from build123d import *

# Parameters (mm, degrees)
SKETCH1_R           = 10.75
BOSS_EXTRUDE1_DEPTH = 7.1
BOSS_EXTRUDE2_DEPTH = 1.5875
SKETCH3_R           = 2.54
BOSS_EXTRUDE3_DEPTH = 29
FILLET1_R           = 1.27


with BuildPart() as part:
    # Sketch1 → Boss-Extrude1 (new body)
    with BuildSketch(Plane(origin=(0, 0, 0), x_dir=(1, 0, 0), z_dir=(0, 1, 0))):
        with Locations(Location((0, 0, 0), (0, 0, 270))):
            Circle(SKETCH1_R)
    extrude(amount=BOSS_EXTRUDE1_DEPTH)

    # Sketch2 → Boss-Extrude2 (add)
    with BuildSketch(Plane.XZ):
        Polygon((-14.837901918, 0), (-7.418950959, -12.85), (7.418950959, -12.85), (14.837901918, 0), (7.418950959, 12.85), (-7.418950959, 12.85), align=None)
    extrude(amount=BOSS_EXTRUDE2_DEPTH)

    # Sketch3 → Boss-Extrude3 (add)
    with BuildSketch(Plane.XZ.offset(1.5875)):
        with Locations(Location((0, 7.80660503, 0), (0, 0, 90))):
            Circle(SKETCH3_R)
        with Locations(Location((0, -7.80660503, 0), (0, 0, 90))):
            Circle(SKETCH3_R)
    extrude(amount=BOSS_EXTRUDE3_DEPTH)

    # Fillet1
    fillet1_edges = [part.edges().sort_by_distance(p)[0] for p in [
        (0, 7.1, -10.75),
    ]]
    fillet(fillet1_edges, radius=FILLET1_R)


solid = part.part
Can you work these out from the model? Positions are in its coordinate system, mm. A direction names the side the tool comes from. Give positions to 0.01 mm unless a question says otherwise; leave off trailing zeros. Order: outer loops, then holes, each group sorted by start corner. A loop starts at its lowest first (then second) coordinate and runs counter-clockwise, first axis right, second up. Notation, with made-up numbers: M 45,60.25 L 70,60.25 A11 ccw 70,77.25 Z; hole C -11.5,67.25 d10. An arc over 180 degrees is marked long. Use one line per item in the form item = value. Start each with the question number.
Item 1: If we section it at B-B (y = -21): Write out the boundary of the cut face in (x, z), then the cut area to 3 significant figures.
Item 2: We'd pull the mould along Z, two halves only. Please class faces 1 (the cylindrical face through (1.55, -15.88, -9.82)), 2 (the flat face through (11.08, -0.78, -6.51)), 3 (the cylindrical face through (7.27, 2.87, -7.92)): +Z half, -Z half, draft (parallel to the pull), parting line (faces both ways), or undercut.
Item 3: Will these pins go through, and if not, where does the flat tip stop? pin 1 Ø1.5 at (y, z) = (-12.5, -10) entering from -X; pin 2 Ø1.5 at (x, z) = (-4.5, -4.5) entering from -Y; pin 3 Ø6 at (y, z) = (-23, 3.5) entering from -X; pin 4 Ø1 at (y, z) = (-14, -3.5) entering from +X.
Item 4: For faces 4 (the cylindrical face through (-1.717, -15.885, 5.935)), 5 (the flat face through (8, 0, 8)), 6 (the flat face through (0, -30.588, -8)), which set-ups out of +Z, -Z, +X, -X, +Y, -Y let a thin tool reach every point of the face, with its end or its side?
Item 5: If we section it at A-A (x = 0): Write out the boundary of the cut face in (y, z).
Item 6: If I drill on line 1 along Y through (x, z) = (11.25, 3.5); line 2 along X through (y, z) = (-12.5, 8); line 3 along Y through (x, z) = (-7.5, 1.75), over which ranges is the centre line in solid material (lowest first)?
Outcome:
q1.outline = C 0,-7.81 d5.08; C 0,7.81 d5.08
q1.area = 40.5 mm2
q2.face_1 = undercut
q2.face_2 = -Z half
q2.face_3 = parting line
q3.pin_1 = -2.09
q3.pin_2 = -1.59
q3.pin_3 = -2.18
q3.pin_4 = through
q4.face_4 = -Y
q4.face_5 = +Y
q4.face_6 = +Z, -Z, +X, -X, -Y
q5.outline = M -30.59,-10.35 L -1.59,-10.35 L -1.59,-12.85 L 0,-12.85 L 0,-10.75 L 5.83,-10.75 A1.27 ccw 7.1,-9.48 L 7.1,9.48 A1.27 ccw 5.83,10.75 L 0,10.75 L 0,12.85 L -1.59,12.85 L -1.59,10.35 L -30.59,10.35 L -30.59,5.27 L -1.59,5.27 L -1.59,-5.27 L -30.59,-5.27 Z
q6.line_1 = -1.59 to 0
q6.line_2 = -2.53 to 2.53
q6.line_3 = -1.59 to 7.1
